```python
from build123d import *

# Parameters (mm, degrees)
SKETCH_W               = 48
SKETCH_H               = 28
PAD_DEPTH              = 4
SKETCH001_W            = 14
SKETCH001_H            = 3
POCKET_DEPTH           = 15
SKETCH002_W            = 4
SKETCH002_H            = 12
SKETCH002_W_2          = 3
SKETCH002_H_2          = 3
POCKET001_DEPTH        = 4.001
SKETCH003_R            = 0.7
PAD001_DEPTH           = 3
FUSION_PLACEMENT_ANGLE = 180


with BuildPart() as pocket001:
    # Sketch → Pad (new body)
    with BuildSketch(Plane.XY):
        with Locations((24, 14)):
            Rectangle(SKETCH_W, SKETCH_H)
    extrude(amount=PAD_DEPTH)

    # Sketch001 → Pocket (cut)
    with BuildSketch(Plane(origin=(0, 0, 0), x_dir=(0, -1, 0), z_dir=(-1, 0, 0))):
        with Locations((-14, 1.5)):
            Rectangle(SKETCH001_W, SKETCH001_H)
    extrude(amount=-POCKET_DEPTH, mode=Mode.SUBTRACT)

    # Sketch002 → Pocket001 (cut, through all)
    with BuildSketch(Plane.XY.offset(4)):
        with Locations((42, 14)):
            Rectangle(SKETCH002_W, SKETCH002_H)
        with Locations((41.5, 6)):
            Rectangle(SKETCH002_W_2, SKETCH002_H_2)
        with Locations((5.5, 5.5)):
            Rectangle(SKETCH002_W_2, SKETCH002_H_2)
        with Locations((5.098741, 22.5)):
            Rectangle(SKETCH002_W_2, SKETCH002_H_2)
    extrude(amount=-POCKET001_DEPTH, mode=Mode.SUBTRACT)


with BuildPart() as fusion:
    # Pad001 base: copy of Pocket001
    add(pocket001.part)

    # Sketch003 → Pad001 (new body)
    with BuildSketch(Plane(origin=(0, 0, 0), x_dir=(1, 0, 0), z_dir=(0, 0, -1))):
        with Locations((1.5, -1.5)):
            Circle(SKETCH003_R)
        with Locations((1.5, -26.5)):
            Circle(SKETCH003_R)
        with Locations((46.109886, -26.5)):
            Circle(SKETCH003_R)
        with Locations((46.109886, -1.5)):
            Circle(SKETCH003_R)
    extrude(amount=PAD001_DEPTH)

    # Fusion: union Pocket001
    add(pocket001.part)


with BuildPart() as fusion_1:
    # Fusion placement: moved
    add(fusion.part.rotate(Axis((0, 0, 0), (0, 1, 0)), FUSION_PLACEMENT_ANGLE))


solid = fusion_1.part
```
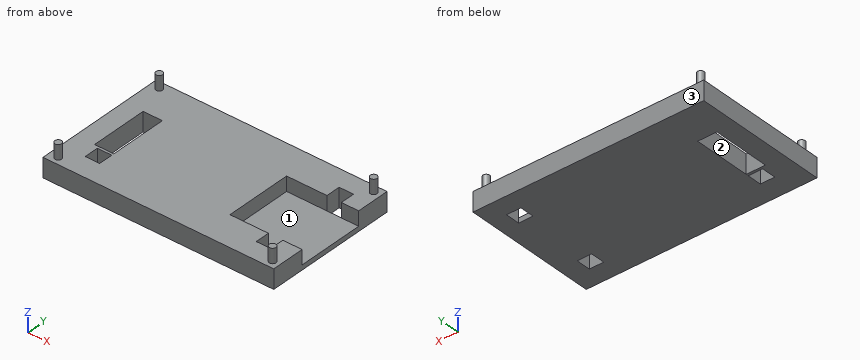
Can you work these out from the model? Positions are in its coordinate system, mm. Face numbers are marked on the shaded views. A direction names the side the tool comes from. Coordinates: 2 decimals unless noted, no trailing zeros. Write each loop counter-clockwise with the first axis right and the second up, starting at its lowest first coordinate (ties: lowest second). Pieces come first, ordered by that corner, then holes. Notation, with made-up numbers: (57, -18) - (113, -18) arc R17 cw to (113, 9) - close; hole circle Ø9 at (25, 52). An arc over 180 degrees is marked (long way). Return JSON: item names as keys, results as strings.
Q1. If we section it at B-B (x = -5): Please give me the cut outline in (y, z).
Computed values:
{"outline": "(0, -4) - (4, -4) - (4, 0) - (0, 0) - close; (7, -4) - (21, -4) - (21, -3) - (7, -3) - close; (24, -4) - (28, -4) - (28, 0) - (24, 0) - close"}
Q2. I'm going to push a flat-ended pin straight in: pin 1 Ø14 at (x, y) = (-31, 20.5) entering from +Z. Where does the tip first touch, or does it pass through?
Computed values:
{"pin 1": "stops at z = 0"}
Q3. If we section it at C-C (y = 26.5): Please give me the cut outline in (x, z), then the cut area to 3 significant figures.
Computed values:
{"outline": "(-48, -4) - (0, -4) - (0, 0) - (-0.8, 0) - (-0.8, 3) - (-2.2, 3) - (-2.2, 0) - (-45.41, 0) - (-45.41, 3) - (-46.81, 3) - (-46.81, 0) - (-48, 0) - close", "area": "200 mm2"}
Q4. On a 3-axis mill with a long thin cutter (end or side, diameter ignored), from which of +Z, -Z, +X, -X, +Y, -Y can I reach the whole of each face in a straight line? I mean the marked faces 1, 2 and 3. Say none if no direction works.
Computed values:
{"face 1": "+Z, +X", "face 2": "+Z, -Z", "face 3": "+Z, -Z, +X, -X, +Y"}
Q5. If we section it at D-D (z = 0.5): Please give me the cut outline in (x, y).
Computed values:
{"outline": "circle Ø1.4 at (-46.11, 1.5); circle Ø1.4 at (-46.11, 26.5); circle Ø1.4 at (-1.5, 1.5); circle Ø1.4 at (-1.5, 26.5)"}
Q6. Please list where these lines run through material, in increasing order: L1, parallel to Y at x = -8.5, z = -1; L2, parallel to Z at x = -44.5, y = 4.25; L3, parallel to X at y = 23.5, z = -1.5. Write a range as from..to.
Computed values:
{"L1": "y = 0..7, 21..28", "L2": "z = -4..0", "L3": "x = -48..-6.6, -3.6..0"}
Q7. If we section it at A-A (y = 15.25): Please give me the cut outline in (x, z).
Computed values:
{"outline": "(-48, -4) - (-44, -4) - (-44, 0) - (-48, 0) - close; (-40, -4) - (0, -4) - (0, -3) - (-15, -3) - (-15, 0) - (-40, 0) - close"}
